Input: part model. Units: mm. Frame: model coordinates. Face numbers are marked on the shaded views. A direction names the side the tool comes from. Round coordinates to 2 decimals unless told otherwise and drop trailing zeros. Write each loop counter-clockwise with the first axis right and the second up, starting at its lowest first coordinate (ties: lowest second). Pieces come first, ordered by that corner, then holes. Notation, with made-up numbers: (51, -35) -> (70, -35) arc R12 cw to (70, -22) -> close; hole circle Ø9 at (-3, -25). An arc over 180 degrees is marked (long way). Write item = value, one per line. Start each with the question number.
```python
from build123d import *

# Parameters (mm, degrees)
BOSS_EXTRUDE1_DEPTH = 229
FILLET1_R           = 20
SKETCH2_W           = 138
SKETCH2_H           = 89
CUT_EXTRUDE1_DEPTH  = 1
FILLET2_R           = 5
SKETCH3_W           = 29
SKETCH3_H           = 77
BOSS_EXTRUDE2_DEPTH = 35
FILLET3_R           = 5
SKETCH4_W           = 38
SKETCH4_H           = 81
BOSS_EXTRUDE3_DEPTH = 39
CUT_EXTRUDE2_REACH  = 323.447
FILLET4_R           = 5
SKETCH6_W           = 26
SKETCH6_H           = 71
BOSS_EXTRUDE4_DEPTH = 46
FILLET5_R           = 5
BOSS_EXTRUDE5_REACH = 299.914
SKETCH7_R           = 4
SKETCH7_R_2         = 5
SKETCH8_W           = 95
SKETCH8_H           = 54
CUT_EXTRUDE3_DEPTH  = 0.5
SKETCH9_R           = 7
BOSS_EXTRUDE6_DEPTH = 7.5
FILLET6_R           = 2


with BuildPart() as part:
    # Sketch1 → Boss-Extrude1 (new body)
    with BuildSketch(Plane(origin=(0, 0, 0), x_dir=(0, 0, -1), z_dir=(1, 0, 0))):
        with BuildLine():
            Line((0, 0), (-185, 0))
            ThreePointArc((-185, 0), (-197.19983645, 9.777135593), (-190.314960072, 23.813761507))
            Line((-190.314960072, 23.813761507), (-92, 70))
            Line((-92, 70), (0, 70))
            Line((0, 70), (0, 0))
        make_face()
    extrude(amount=BOSS_EXTRUDE1_DEPTH)

    # Fillet1
    fillet1_edges = [part.edges().sort_by_distance(p)[0] for p in [
        (114.5, 70, 92),
    ]]
    fillet(fillet1_edges, radius=FILLET1_R)

    # Sketch2 → Cut-Extrude1 (cut)
    with BuildSketch(Plane(origin=(0, 92.750371214, 43.572115191), x_dir=(1, 0, 0), z_dir=(0, 0.9051009205620354, 0.42519680572383906))):
        with Locations((114.5, -110.048995253)):
            Rectangle(SKETCH2_W, SKETCH2_H)
    extrude(amount=-CUT_EXTRUDE1_DEPTH, mode=Mode.SUBTRACT)

    # Fillet2
    fillet2_edges = [part.edges().sort_by_distance(p)[0] for p in [
        (45.5, 26.584081644, 183.241954664),
        (45.5, 64.426597354, 102.687972734),
        (183.5, 64.426597354, 102.687972734),
        (183.5, 26.584081644, 183.241954664),
    ]]
    fillet(fillet2_edges, radius=FILLET2_R)

    # Sketch3 → Boss-Extrude2 (add)
    with BuildSketch(Plane(origin=(0, 70, 0), x_dir=(1, 0, 0), z_dir=(0, 1, 0))):
        with Locations((15, -43.768114008)):
            Rectangle(SKETCH3_W, SKETCH3_H)
    extrude(amount=BOSS_EXTRUDE2_DEPTH)

    # Fillet3
    fillet3_edges = [part.edges().sort_by_distance(p)[0] for p in [
        (15, 105, 5.268114008),
        (15, 105, 82.268114008),
    ]]
    fillet(fillet3_edges, radius=FILLET3_R)

    # Sketch4 → Boss-Extrude3 (add)
    with BuildSketch(Plane(origin=(0, 70, 0), x_dir=(1, 0, 0), z_dir=(0, 1, 0))):
        with Locations((209.5, -43.768114008)):
            Rectangle(SKETCH4_W, SKETCH4_H)
    extrude(amount=BOSS_EXTRUDE3_DEPTH)

    # Sketch5 → Cut-Extrude2 (cut, up to next)
    with BuildSketch(Plane(origin=(229, 0, 0), x_dir=(0, 0, -1), z_dir=(1, 0, 0)), mode=Mode.PRIVATE) as cut_extrude2_sk1:
        Polygon((-62.768114008, 109), (-43.768114008, 90), (-24.768114008, 109), align=None)
    cut_extrude2_tool1 = extrude(cut_extrude2_sk1.sketch, amount=-CUT_EXTRUDE2_REACH, mode=Mode.PRIVATE) & part.part
    add(cut_extrude2_tool1.solids().sort_by_distance((229, 102.666667, 43.768114))[0], mode=Mode.SUBTRACT)

    # Fillet4
    fillet4_edges = [part.edges().sort_by_distance(p)[0] for p in [
        (209.5, 90, 43.768114008),
        (209.5, 109, 24.768114008),
        (209.5, 109, 62.768114008),
        (209.5, 109, 3.268114008),
        (209.5, 109, 84.268114008),
    ]]
    fillet(fillet4_edges, radius=FILLET4_R)

    # Sketch6 → Boss-Extrude4 (add)
    with BuildSketch(Plane(origin=(0, 70, 0), x_dir=(1, 0, 0), z_dir=(0, 1, 0))):
        with Locations((90.5, -43.768114008)):
            Rectangle(SKETCH6_W, SKETCH6_H)
    extrude(amount=BOSS_EXTRUDE4_DEPTH)

    # Fillet5
    fillet5_edges = [part.edges().sort_by_distance(p)[0] for p in [
        (90.5, 116, 8.268114008),
        (90.5, 116, 79.268114008),
    ]]
    fillet(fillet5_edges, radius=FILLET5_R)

    # Boss-Extrude5: up to this face of the body (flat: up to its plane)
    boss_extrude5_end = Plane(part.part.faces().sort_by_distance((29.5, 87.434510008, 43.768114008))[0])
    # Sketch7 → Boss-Extrude5 (add, up to the picked face)
    with BuildSketch(Plane.ZY.offset(-190.5), mode=Mode.PRIVATE) as boss_extrude5_sk1:
        with Locations(Location((14.768114008, 78, 0), (0, 0, 180))):
            Circle(SKETCH7_R)
    boss_extrude5_tool1 = split(extrude(boss_extrude5_sk1.sketch, amount=BOSS_EXTRUDE5_REACH, mode=Mode.PRIVATE), bisect_by=boss_extrude5_end, keep=Keep.BOTH, mode=Mode.PRIVATE)
    # Sketch7 → Boss-Extrude5 (add, up to the picked face)
    with BuildSketch(Plane.ZY.offset(-190.5), mode=Mode.PRIVATE) as boss_extrude5_sk2:
        with Locations(Location((43.768114008, 78, 0), (0, 0, 180))):
            Circle(SKETCH7_R_2)
    boss_extrude5_tool2 = split(extrude(boss_extrude5_sk2.sketch, amount=BOSS_EXTRUDE5_REACH, mode=Mode.PRIVATE), bisect_by=boss_extrude5_end, keep=Keep.BOTH, mode=Mode.PRIVATE)
    # Sketch7 → Boss-Extrude5 (add, up to the picked face)
    with BuildSketch(Plane.ZY.offset(-190.5), mode=Mode.PRIVATE) as boss_extrude5_sk3:
        with Locations(Location((72.768114008, 78, 0), (0, 0, 180))):
            Circle(SKETCH7_R)
    boss_extrude5_tool3 = split(extrude(boss_extrude5_sk3.sketch, amount=BOSS_EXTRUDE5_REACH, mode=Mode.PRIVATE), bisect_by=boss_extrude5_end, keep=Keep.BOTH, mode=Mode.PRIVATE)
    add(boss_extrude5_tool1.solids().sort_by(Axis((190.5, 78, 14.768114), (-1, 0, 0)))[0])
    add(boss_extrude5_tool2.solids().sort_by(Axis((190.5, 78, 43.768114), (-1, 0, 0)))[0])
    add(boss_extrude5_tool3.solids().sort_by(Axis((190.5, 78, 72.768114), (-1, 0, 0)))[0])

    # Sketch8 → Cut-Extrude3 (cut)
    with BuildSketch(Plane(origin=(0, 91.845270293, 43.146918385), x_dir=(1, 0, 0), z_dir=(0, 0.9051009205620354, 0.425196805723839))):
        with Locations((114.5, -110.048995253)):
            Rectangle(SKETCH8_W, SKETCH8_H)
    extrude(amount=-CUT_EXTRUDE3_DEPTH, mode=Mode.SUBTRACT)

    # Sketch9 → Boss-Extrude6 (add)
    with BuildSketch(Plane(origin=(0, 0, 0), x_dir=(-1, 0, 0), z_dir=(0, -1, 0))):
        with Locations(Location((-11, -171, 0), (0, 0, 270))):
            Circle(SKETCH9_R)
        with Locations(Location((-11, -14, 0), (0, 0, 270))):
            Circle(SKETCH9_R)
        with Locations(Location((-218, -171, 0), (0, 0, 270))):
            Circle(SKETCH9_R)
        with Locations(Location((-218, -14, 0), (0, 0, 270))):
            Circle(SKETCH9_R)
    extrude(amount=BOSS_EXTRUDE6_DEPTH)

    # Fillet6
    fillet6_edges = [part.edges().sort_by_distance(p)[0] for p in [
        (218, -7.5, 7),
        (218, -7.5, 164),
        (11, -7.5, 164),
        (11, -7.5, 7),
    ]]
    fillet(fillet6_edges, radius=FILLET6_R)


solid = part.part
```
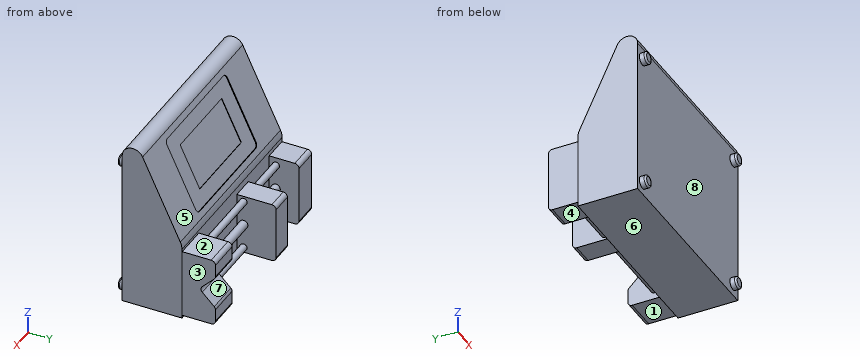
1. Section B-B (x = 93). Output: boundary loops of the cut face in (y, z).
2. Line query: line 1 along X through (y, z) = (88.5, 59); line 2 along Z through (x, y) = (120, 80); line 3 along Z through (x, y) = (161, 77). Output: solid intervals per line, ascending.
3. Reachability of the marked faces 1, 2, 3 and 4 from +Z, -Z, +X, -X, +Y, -Y: full face, straight path, thin tool, end or side. Return the list, or none.
4. Section D-D (x = 138.5). Output: boundary loops of the cut face in (y, z).
5. Section C-C (z = 146). Output: boundary loops of the cut face in (x, y), then the cut area to 3 significant figures.
6. Pin query (flat end, axial travel): P1, Ø23, axis at y = 101.5, z = 33, coming from the +X side; P2, Ø6, axis at x = 143.5, y = 18, coming from the +Z side; P3, Ø23, axis at y = 90.5, z = 54.5, coming from the -X side; P4, Ø7, axis at y = 40.5, z = 144, coming from the -X side. Return the tip coordinate at first contact, or that it passes through.
7. Section A-A (x = 55). Output: boundary loops of the cut face in (y, z), then the cut area to 3 significant figures.
8. Mould query, pull axis Z, two halves, no side actions, for the marked faces 5, 6, 7 and 8. Classes: pulls with the +Z half, pulls with the -Z half, needs draft (parallel to the pull), parting line crosses it, or undercut.
Check sheet entries:
q1.outline = (0, 0) -> (70, 0) -> (70, 8.27) -> (111, 8.27) arc R5 ccw to (116, 13.27) -> (116, 74.27) arc R5 ccw to (111, 79.27) -> (70, 79.27) -> (70, 87.54) arc R20 ccw to (68.1, 96.04) -> (64.88, 102.9) -> (63.97, 102.48) -> (56.53, 118.31) -> (56.08, 118.1) -> (33.12, 166.98) -> (33.57, 167.19) -> (26.13, 183.03) -> (27.04, 183.45) -> (23.81, 190.31) arc R12.5 ccw to (0, 185) -> close
q2.line_1 = 0.5 to 29.5, 77.5 to 103.5, 190.5 to 228.5
q2.line_2 = 11.3 to 18.23, 39.19 to 48.35, 69.3 to 76.23
q2.line_3 = 10.9 to 18.64, 38.87 to 48.67, 68.9 to 76.64
q3.face_1 = -Z, +X, -X, +Y
q3.face_2 = +Z, +X, -X, +Y
q3.face_3 = +Z, -Z, +X, +Y
q3.face_4 = -Z, -X, +Y
q4.outline = (0, 0) -> (70, 0) -> (70, 87.54) arc R20 ccw to (68.1, 96.04) -> (64.88, 102.9) -> (63.97, 102.48) -> (56.53, 118.31) -> (56.08, 118.1) -> (33.12, 166.98) -> (33.57, 167.19) -> (26.13, 183.03) -> (27.04, 183.45) -> (23.81, 190.31) arc R12.5 ccw to (0, 185) -> close; circle Ø10 at (78, 43.77); circle Ø8 at (78, 14.77); circle Ø8 at (78, 72.77)
q5.outline = (0, 0) -> (229, 0) -> (229, 44.63) -> (183.5, 44.63) -> (183.5, 43.53) -> (162, 43.53) -> (162, 42.97) -> (67, 42.97) -> (67, 43.53) -> (45.5, 43.53) -> (45.5, 44.63) -> (0, 44.63) -> close
q5.area = 10,000 mm2
q6.P1 = 228.5
q6.P2 = 197.25
q6.P3 = 0.5
q6.P4 = 0
q7.outline = (0, 0) -> (70, 0) -> (70, 87.54) arc R20 ccw to (68.1, 96.04) -> (64.88, 102.9) -> (63.97, 102.48) -> (26.13, 183.03) -> (27.04, 183.45) -> (23.81, 190.31) arc R12.5 ccw to (0, 185) -> close; circle Ø10 at (78, 43.77); circle Ø8 at (78, 14.77); circle Ø8 at (78, 72.77)
q7.area = 11,300 mm2
q8.face_5 = pulls with the +Z half
q8.face_6 = pulls with the -Z half
q8.face_7 = undercut
q8.face_8 = undercut
